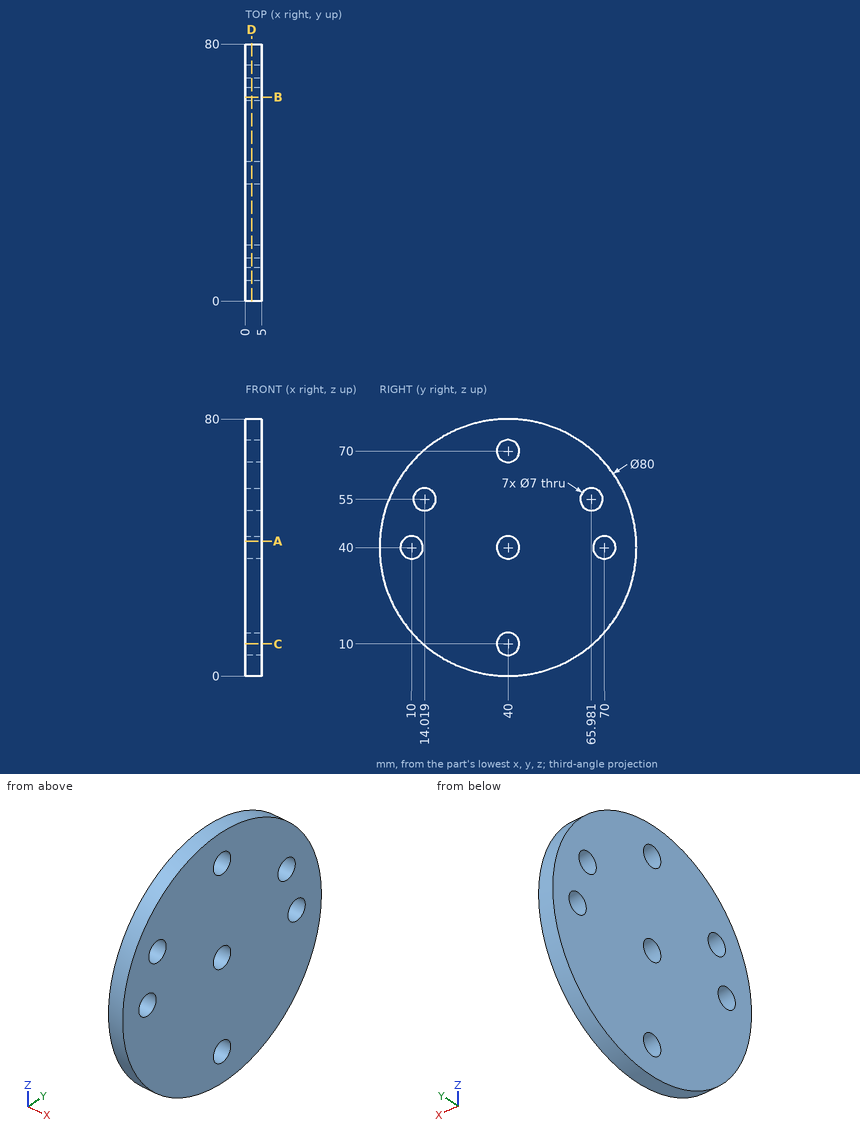
Check sheet for the drawn part. Datum: minimum x, y, z corner. Units: mm. Round coordinates to 2 decimals unless told otherwise and drop trailing zeros. Order: outer loops, then holes, each group sorted by start corner. A loop starts at its lowest first (then second) coordinate and runs counter-clockwise, first axis right, second up. Notation, with made-up numbers: (-18.75, 22) -> (40.25, 22) arc R22 cw to (40.25, 30) -> close; hole circle Ø5 at (-15.75, -18). An arc over 180 degrees is marked (long way). Put each result on its own line as item: value. Start each with the question number.
(1) Section check B-B (y = 63.5). Enter the section's corners in (x, z), then the cut area to 3 significant figures.
(2) Section check D-D (x = 1.9). Enter the section's corners in (y, z), then the cut area to 3 significant figures.
(3) Material ranges on line 1 along Y through (x, z) = (1.85, 55); line 2 along Z through (x, y) = (4.6, 67.5); line 3 along Y through (x, z) = (2.5, 70), recorded low to high.
(4) Section check A-A (z = 42). Enter the section's corners in (x, y), then the cut area to 3 significant figures.
(5) Section check C-C (z = 10). Enter the section's corners in (x, y), then the cut area to 3 significant figures.
Completed:
1. outline: (0, 7.63) -> (5, 7.63) -> (5, 52.53) -> (0, 52.53) -> close; (0, 57.47) -> (5, 57.47) -> (5, 72.37) -> (0, 72.37) -> close
1. area: 299 mm2
2. outline: circle Ø80 at (40, 40); hole circle Ø7 at (10, 40); hole circle Ø7 at (14.02, 55); hole circle Ø7 at (40, 10); hole circle Ø7 at (40, 40); hole circle Ø7 at (40, 70); hole circle Ø7 at (65.98, 55); hole circle Ø7 at (70, 40)
2. area: 4,760 mm2
3. line 1: y = 2.92 to 10.52, 17.52 to 62.48, 69.48 to 77.08
3. line 2: z = 10.95 to 37.55, 42.45 to 51.85, 58.15 to 69.05
3. line 3: y = 13.54 to 36.5, 43.5 to 66.46
4. outline: (0, 0.05) -> (5, 0.05) -> (5, 7.13) -> (0, 7.13) -> close; (0, 12.87) -> (5, 12.87) -> (5, 37.13) -> (0, 37.13) -> close; (0, 42.87) -> (5, 42.87) -> (5, 67.13) -> (0, 67.13) -> close; (0, 72.87) -> (5, 72.87) -> (5, 79.95) -> (0, 79.95) -> close
4. area: 313 mm2
5. outline: (0, 13.54) -> (5, 13.54) -> (5, 36.5) -> (0, 36.5) -> close; (0, 43.5) -> (5, 43.5) -> (5, 66.46) -> (0, 66.46) -> close
5. area: 230 mm2
